Part model, mm, in its own coordinate system. A direction names the side the tool comes from. Give positions to 0.01 mm unless a question says otherwise; leave off trailing zeros. Write each loop counter-clockwise with the first axis right and the second up, starting at its lowest first coordinate (ties: lowest second). Pieces come first, ordered by that corner, then holes.
from build123d import *

# Parameters (mm, degrees)
SKETCH_1_W          = 78
SKETCH_1_H          = 50
EXTRUDE_1_DEPTH     = 2
SKETCH_2_R          = 6
SKETCH_2_R_2        = 4
CUT_EXTRUDE_2_DEPTH = 3
CUT_EXTRUDE_3_DEPTH = 3


with BuildPart() as part:
    # Эскиз1 → Бобышка-Вытянуть1 (new body)
    with BuildSketch(Plane.XY):
        with Locations((-7, 7)):
            Rectangle(SKETCH_1_W, SKETCH_1_H)
    extrude(amount=EXTRUDE_1_DEPTH)

    # Эскиз2 → Вырез-Вытянуть2 (cut, through all)
    with BuildSketch(Plane.XY.offset(2)):
        with Locations((-32.5, 18)):
            Circle(SKETCH_2_R)
        with Locations((-20, 18)):
            Circle(SKETCH_2_R)
        with Locations((0, 18)):
            Circle(SKETCH_2_R)
        with Locations((15, 18)):
            Circle(SKETCH_2_R)
        with Locations((-14, -8)):
            Circle(SKETCH_2_R_2)
        with Locations((-31.749315539, -5.262317493)):
            Circle(SKETCH_2_R)
    extrude(amount=-CUT_EXTRUDE_2_DEPTH, mode=Mode.SUBTRACT)

    # Эскиз3 → Вырез-Вытянуть3 (cut, through all)
    with BuildSketch(Plane.XY.offset(2)):
        Polygon((-37.708738379, -4.565697495), (-39.23827254, -18), (-22.345634052, -18), (-25.7898927, -4.565697495), align=None)
        Polygon((-16.128623671, -11.386585488), (-16.128623671, -18), (-11.733531884, -18), (-11.733531884, -11.295925102), align=None)
        Polygon((-40.319551463, 32), (-38.5, 18), (-32.5, 12), (-20, 12), (-14, 18), (-13.221505596, 32), align=None)
        Polygon((-8.134373627, 32), (-5.917388606, 17.007774179), (-0.949072404, 12.075537022), (15.949072404, 12.075537022), (20.784965527, 16.40809113), (23.68000723, 32), align=None)
    extrude(amount=-CUT_EXTRUDE_3_DEPTH, mode=Mode.SUBTRACT)


solid = part.part
1) Saw through at A-A (y = 15). Write the cut outline in (x, z).
Check result:
outline: (-46, 0) - (-37.7, 0) - (-37.7, 2) - (-46, 2) - close; (-14.8, 0) - (-5.2, 0) - (-5.2, 2) - (-14.8, 2) - close; (20.2, 0) - (32, 0) - (32, 2) - (20.2, 2) - close
2) Saw through at D-D (x = 19). Write the cut outline in (y, z), and give its area (3 significant figures).
Check result:
outline: (-18, 0) - (13.53, 0) - (13.53, 2) - (-18, 2) - close
area: 63.1 mm2
3) 3-axis set-ups, long thin cutter, end or side, ignore diameter. For faces 4 (the flat face through (-11.734, -15, 1)), 5 (the cylindrical face through (-15.804, 13.711, 1.014)), 6 (the flat face through (28, 32, 1)): which of +Z, -Z, +X, -X, +Y, -Y reach the whole face in a straight line?
Check result:
face 4: +Z, -Z, -Y
face 5: +Z, -Z, +Y
face 6: +Z, -Z, +X, -X, +Y
4) Saw through at C-C (y = -13.5). Write the cut outline in (x, z), and give its area (3 significant figures).
Check result:
outline: (-46, 0) - (-38.73, 0) - (-38.73, 2) - (-46, 2) - close; (-23.5, 0) - (-16.13, 0) - (-16.13, 2) - (-23.5, 2) - close; (-11.73, 0) - (32, 0) - (32, 2) - (-11.73, 2) - close
area: 117 mm2
5) Flat gauge pins, fed straight in: P1, Ø1, axis at x = -34, z = 1, coming from the +Y side; P2, Ø0.6, axis at x = -26, z = 1.5, coming from the +Y side; P3, Ø7, axis at x = -14, y = -8, coming from the -Z side. Where does each tip first touch, or does it go through?
Check result:
P1: stops at y = 12.34
P2: stops at y = 12
P3: passes through
6) Saw through at B-B (z = 0.4). Write the cut outline in (x, y), and give its area (3 significant figures).
Check result:
outline: (-46, -18) - (-39.24, -18) - (-37.71, -4.6) arc R6 cw to (-25.79, -4.57) - (-22.35, -18) - (-16.13, -18) - (-16.13, -11.39) arc R4 cw (long way) to (-11.73, -11.3) - (-11.73, -18) - (32, -18) - (32, 32) - (23.68, 32) - (20.97, 17.41) arc R6 cw to (14.05, 12.08) - (0.95, 12.08) arc R6 cw to (-5.95, 17.24) - (-8.13, 32) - (-13.22, 32) - (-14, 18) arc R6 cw to (-20, 12) - (-32.5, 12) arc R6 cw to (-38.5, 18) - (-40.32, 32) - (-46, 32) - close
area: 2,530 mm2
7) Mould opens along X. For faces 1 (the flat face through (-11, 32, 1)), 2 (the flat face through (-38.465, -11.207, 1.014)), 3 (the flat face through (-46, 7, 1)) say: +X half, -X half, draft (parallel to the pull), parting line (faces both ways), or undercut.
Check result:
face 1: draft
face 2: undercut
face 3: -X half
8) Drill centre lines: L1, parallel to X at y = 16.5, z = 0.85; L2, parallel to X at y = 28, z = 1.3; L3, parallel to Y at x = -21, z = 1.1. Where is each one in solid material? Low to high.
Check result:
L1: x = -46 to -38.31, -14.19 to -5.81, 20.81 to 32
L2: x = -46 to -39.8, -13.44 to -7.54, 22.94 to 32
L3: y = -18 to 12
